Work out the finished part from the listing and answer in its coordinate system (mm). A direction names the side the tool comes from. Coordinates: 2 decimals unless noted, no trailing zeros. Loops run counter-clockwise (first coordinate to the right, second up) from the corner with the lowest first, then second, coordinate; pieces in that order, holes last.
```python
from build123d import *

# Parameters (mm, degrees)
SKETCH1_W           = 203.2
SKETCH1_H           = 203.2
BOSS_EXTRUDE1_DEPTH = 3.175
CUT_EXTRUDE4_DEPTH  = 144.719172782


with BuildPart() as part:
    # Sketch1 → Boss-Extrude1 (new body)
    with BuildSketch(Plane.XY):
        Rectangle(SKETCH1_W, SKETCH1_H)
    extrude(amount=-BOSS_EXTRUDE1_DEPTH)

    # Sketch10 → Cut-Extrude4 (cut, through all)
    with BuildSketch(Plane.XY):
        with BuildLine():
            Line((96.8375, 42.814327494), (80.9625, 33.648891971))
            ThreePointArc((80.9625, 33.648891971), (77.476108029, 30.1625), (76.2, 25.4))
            Line((76.2, 25.4), (76.2, -25.4))
            ThreePointArc((76.2, -25.4), (77.476108029, -30.1625), (80.9625, -33.648891971))
            Line((80.9625, -33.648891971), (96.8375, -42.814327494))
            ThreePointArc((96.8375, -42.814327494), (100.323891971, -46.300719465), (101.6, -51.063219465))
            Line((101.6, -51.063219465), (101.6, 51.063219465))
            ThreePointArc((101.6, 51.063219465), (100.323891971, 46.300719465), (96.8375, 42.814327494))
        make_face()
    extrude(amount=-CUT_EXTRUDE4_DEPTH, mode=Mode.SUBTRACT)


solid = part.part
```
1. Straight lines are drawn through the part: probe 1 along Y at (x, z) = (77.5, -1.95); probe 2 along X at (y, z) = (-24, -1.05); probe 3 along X at (y, z) = (-49.5, -2.45). For each, find the intervals that lie inside material, in ascending order.
2. For faces 3 (the flat face through (-1, 1, -3.175)), 4 (the cylindrical face through (100.29, -46.24, -1.57)), determine the directions among +Z, -Z, +X, -X, +Y, -Y from which every point of the face is accessible in a straight line to the end or side of a thin tool.
3. A cutting plane is placed at B-B, the plane y = 1.5. Give the vertices of the cut face in (x, z) (3 decimals), then the cut area to 3 significant figures.
4. Determine the mould class of faces 1 (the flat face through (-1, 1, 0)), 2 (the cylindrical face through (77.44, -30.1, -1.57)) for opening direction Y: released by +Y, released by -Y, zero draft, split by the parting line, or undercut.
5. A cutting plane is placed at C-C, the plane y = 37. Give the vertices of the cut face in (x, z) (3 decimals), then the cut area to 3 significant figures.
Answers below:
1. probe 1: y = -101.6 to -30.2, 30.2 to 101.6
1. probe 2: x = -101.6 to 76.2
1. probe 3: x = -101.6 to 101.47
2. face 3: -Z, +X, -X, +Y, -Y
2. face 4: +Z, -Z, +X
3. outline: (-101.6, -3.175) - (76.2, -3.175) - (76.2, 0) - (-101.6, 0) - close
3. area: 565 mm2
4. face 1: zero draft
4. face 2: undercut
5. outline: (-101.6, -3.175) - (86.767, -3.175) - (86.767, 0) - (-101.6, 0) - close
5. area: 598 mm2
